Design review of the part built by this model. Coordinates are the model's own, in mm. Coordinates: 2 decimals unless noted, no trailing zeros. Write each loop counter-clockwise with the first axis right and the second up, starting at its lowest first coordinate (ties: lowest second). Pieces come first, ordered by that corner, then holes. Notation, with made-up numbers: M 15,2 L 29,2 A26 cw 29,30 Z; hole C -22.5,26 d10. An arc over 180 degrees is marked long. Write item = value, one per line.
```python
from build123d import *

# Parameters (mm, degrees)
SKETCH2_W           = 20
SKETCH2_H           = 20
BOSS_EXTRUDE1_DEPTH = 5
SKETCH3_R           = 1.6
CUT_EXTRUDE1_DEPTH  = 6
FILLET1_R           = 2


with BuildPart() as part:
    # Sketch2 → Boss-Extrude1 (new body)
    with BuildSketch(Plane(origin=(0, 0, 0), x_dir=(1, 0, 0), z_dir=(0, 1, 0))):
        with Locations((10, 10)):
            Rectangle(SKETCH2_W, SKETCH2_H)
    extrude(amount=BOSS_EXTRUDE1_DEPTH)

    # Sketch3 → Cut-Extrude1 (cut, through all)
    with BuildSketch(Plane(origin=(0, 5, 0), x_dir=(1, 0, 0), z_dir=(0, 1, 0))):
        with Locations((10, 10)):
            Circle(SKETCH3_R)
    extrude(amount=-CUT_EXTRUDE1_DEPTH, mode=Mode.SUBTRACT)

    # Fillet1
    fillet1_edges = [part.edges().sort_by_distance(p)[0] for p in [
        (10, 5, -20),
        (0, 5, -10),
        (10, 5, 0),
        (0, 2.5, 0),
        (0, 2.5, -20),
        (20, 2.5, -20),
        (20, 2.5, 0),
        (20, 5, -10),
    ]]
    fillet(fillet1_edges, radius=FILLET1_R)


solid = part.part
```
Q1. The part is to be moulded in two halves that separate along X. For faces 1 (the cylindrical face through (0.57, 1.52, -0.6)), 2 (the cylindrical face through (8.4, 2.54, -10.07)), 3 (the cylindrical face through (19.4, 1.52, -0.57)), 4 (the cylindrical face through (10.11, 4.4, -0.57)), say which applies: +X half, -X half, draft (parallel to the pull), parting line (faces both ways), or undercut.
Check result:
face_1 = -X half
face_2 = undercut
face_3 = +X half
face_4 = draft
Q2. Consider section B-B, the plane y = 0.5. State the section outline as (x, z) points, and give its area (3 significant figures).
Check result:
outline = M 0,-18 A2 ccw 2,-20 L 18,-20 A2 ccw 20,-18 L 20,-2 A2 ccw 18,0 L 2,0 A2 ccw 0,-2 Z; hole C 10,-10 d3.2
area = 389 mm²
Q3. Consider section A-A, the plane z = -10. State the section outline as (x, y) points.
Check result:
outline = M 0,0 L 8.4,0 L 8.4,5 L 2,5 A2 ccw 0,3 Z; M 11.6,0 L 20,0 L 20,3 A2 ccw 18,5 L 11.6,5 Z
Q4. Wall thickness on line 1 (X direction, y = 1, z = -10); line 2 (Z direction, x = 10, y = 2.15); line 3 (Z direction, x = 3.75, y = 4.65): over which ranges is each line inside the solid? List them lowest first.
Check result:
line_1 = 0 to 8.4, 11.6 to 20
line_2 = -20 to -11.6, -8.4 to 0
line_3 = -19.13 to -0.87
Q5. Consider section C-C, the plane x = 10. State the section outline as (y, z) points.
Check result:
outline = M 0,-20 L 3,-20 A2 ccw 5,-18 L 5,-11.6 L 0,-11.6 Z; M 0,-8.4 L 5,-8.4 L 5,-2 A2 ccw 3,0 L 0,0 Z
Q6. Consider section D-D, the plane z = -6. State the section outline as (x, y) points.
Check result:
outline = M 0,0 L 20,0 L 20,3 A2 ccw 18,5 L 2,5 A2 ccw 0,3 Z
